Can you work these out from the model? Positions are in its coordinate system, mm. A direction names the side the tool comes from. Give positions to 0.01 mm unless a question says otherwise; leave off trailing zeros. Order: outer loops, then holes, each group sorted by start corner. A loop starts at its lowest first (then second) coordinate and runs counter-clockwise, first axis right, second up. Notation, with made-up numbers: M 59,64.25 L 92,64.25 A14 cw 92,91.25 Z; hole C -13,86.5 d5. An arc over 180 degrees is marked long. Use a Markdown table: item, result. Add a question column.
from build123d import *

# Parameters (mm, degrees)
BOSS_EXTRUDE1_DEPTH = 10
SKETCH6_R           = 1.6
CUT_EXTRUDE1_DEPTH  = 10
SKETCH7_R           = 1.6
CUT_EXTRUDE2_DEPTH  = 10
SKETCH9_R           = 2.6
CUT_EXTRUDE4_DEPTH  = 10


with BuildPart() as part:
    # Sketch1 → Boss-Extrude1 (new body)
    with BuildSketch(Plane.XY):
        Polygon((-35, 0), (35, 0), (35, -25), (20, -25), (20, -65), (-20, -65), (-20, -25), (-35, -25), align=None)
    extrude(amount=BOSS_EXTRUDE1_DEPTH)

    # Sketch6 → Cut-Extrude1 (cut)
    with BuildSketch(Plane(origin=(0, 0, 0), x_dir=(-1, 0, 0), z_dir=(0, 0, -1))):
        with Locations((10, -55)):
            Circle(SKETCH6_R)
        with Locations((-10, -55)):
            Circle(SKETCH6_R)
    extrude(amount=-CUT_EXTRUDE1_DEPTH, mode=Mode.SUBTRACT)

    # Sketch7 → Cut-Extrude2 (cut)
    with BuildSketch(Plane(origin=(0, 0, 0), x_dir=(-1, 0, 0), z_dir=(0, 0, -1))):
        with Locations((0, -31.3)):
            Circle(SKETCH7_R)
    extrude(amount=-CUT_EXTRUDE2_DEPTH, mode=Mode.SUBTRACT)

    # Sketch9 → Cut-Extrude4 (cut)
    with BuildSketch(Plane.XY.offset(10)):
        with Locations((-25, -12.5)):
            Circle(SKETCH9_R)
        with Locations((25, -12.5)):
            Circle(SKETCH9_R)
    extrude(amount=-CUT_EXTRUDE4_DEPTH, mode=Mode.SUBTRACT)


solid = part.part
1. I need wall thicknesses on L1, parallel to Y at x = -10, z = 1; L2, parallel to Y at x = -25, z = 5.75; L3, parallel to X at y = -13, z = 9.25. Which ranges of each line are inside material? Lowest first, please. Write a range as [from, to].
2. On a 3-axis mill with a long thin cutter (end or side, diameter ignored), from which of +Z, -Z, +X, -X, +Y, -Y can I reach the whole of each face in a straight line? I mean faces 1 (the face through (35, -12, 5)), 2 (the face through (20, -45, 5)), 3 (the face through (-20, -45, 5)). Say none if no direction works.
3. If we section it at B-B, the plane x = 10: List the corners of the cut face in (y, z) for me.
4. If we section it at C-C, the plane z = 6: List the corners of the cut face in (x, y) for me.
5. If we section it at D-D, the plane y = -31.3: List the corners of the cut face in (x, z) for me, then the cut area to 3 significant figures.
6. Will these pins go through, and if not, where does the flat tip stop? pin 1 (3 mm diameter, centred on y = -55, z = 6, fed in from -X); pin 2 (3 mm diameter, centred on x = -24.5, z = 4, fed in from -Y).
7. If we section it at A-A, the plane y = -55: List the corners of the cut face in (x, z) for me, then the cut area to 3 significant figures.
Geometry results:
| question | item | result |
|---|---|---|
| 1 | L1 | y = [-65, -56.6], [-53.4, 0] |
| 1 | L2 | y = [-25, -15.1], [-9.9, 0] |
| 1 | L3 | x = [-35, -27.55], [-22.45, 22.45], [27.55, 35] |
| 2 | face 1 | +Z, -Z, +X, +Y, -Y |
| 2 | face 2 | +Z, -Z, +X, -Y |
| 2 | face 3 | +Z, -Z, -X, -Y |
| 3 | outline | M -65,0 L -56.6,0 L -56.6,10 L -65,10 Z; M -53.4,0 L 0,0 L 0,10 L -53.4,10 Z |
| 4 | outline | M -35,-25 L -20,-25 L -20,-65 L 20,-65 L 20,-25 L 35,-25 L 35,0 L -35,0 Z; hole C -25,-12.5 d5.2; hole C -10,-55 d3.2; hole C 0,-31.3 d3.2; hole C 10,-55 d3.2; hole C 25,-12.5 d5.2 |
| 5 | outline | M -20,0 L -1.6,0 L -1.6,10 L -20,10 Z; M 1.6,0 L 20,0 L 20,10 L 1.6,10 Z |
| 5 | area | 368 mm^2 |
| 6 | pin 1 | stops at x = -20 |
| 6 | pin 2 | stops at y = -25 |
| 7 | outline | M -20,0 L -11.6,0 L -11.6,10 L -20,10 Z; M -8.4,0 L 8.4,0 L 8.4,10 L -8.4,10 Z; M 11.6,0 L 20,0 L 20,10 L 11.6,10 Z |
| 7 | area | 336 mm^2 |
